The drawing under review shows one solid part. Ordinate dimensions are in mm from its lowest x, y, z. Give positions to 0.01 mm unless a question says otherwise; leave off trailing zeros. Order: outer loops, then holes, each group sorted by start corner. A loop starts at its lowest first (then second) coordinate and runs counter-clockwise, first axis right, second up. Notation, with made-up numbers: (44.25, -21) -> (71.25, -21) arc R32 cw to (71.25, 5) -> close; hole circle Ø11 at (-1.5, 56.5). An arc over 180 degrees is marked (long way). Use CSV: the item, a comma, the result in double quotes. Start each with the question number.
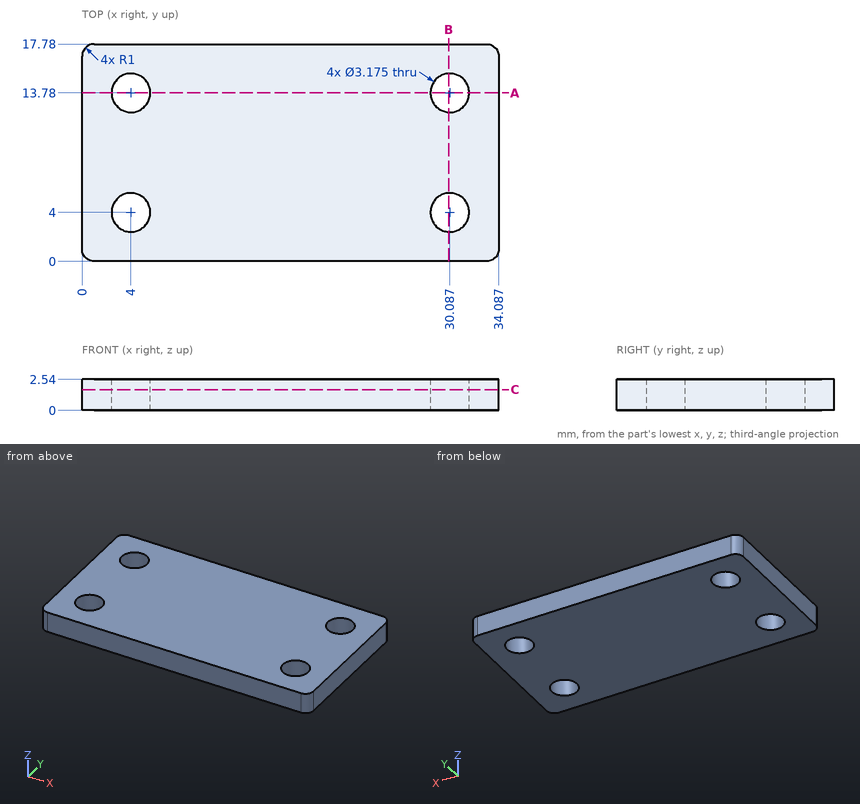
1. To check wall thickness, follow L1, parallel to Y at x = 4, z = 1.5; L2, parallel to Y at x = 5, z = 0.1. State the ranges of each line that lie inside material, in increasing order. Write a range as [from, to].
2. Consider section C-C (z = 1.7). State the section outline as (x, y) points (1 decimal).
3. Consider section A-A (y = 13.78). State the section outline as (x, z) points.
4. Consider section B-B (x = 30). State the section outline as (y, z) points (1 decimal).
5. Clearance check with flat-ended pins moving along their axes: P1, Ø4, axis at x = 4, y = 4, coming from the +Z side; P2, Ø3, axis at x = 30.09, y = 4, coming from the -Z side. State where each tip first meets the part, or that it passes through.
Answer list:
1,L1,"[0, 2.41], [5.59, 12.19], [15.37, 17.78]"
1,L2,"[0, 2.77], [5.23, 12.55], [15.01, 17.78]"
2,outline,"(0, 1) arc R1 ccw to (1, 0) -> (33.1, 0) arc R1 ccw to (34.1, 1) -> (34.1, 16.8) arc R1 ccw to (33.1, 17.8) -> (1, 17.8) arc R1 ccw to (0, 16.8) -> close; hole circle Ø3.2 at (4, 4); hole circle Ø3.2 at (4, 13.8); hole circle Ø3.2 at (30.1, 4); hole circle Ø3.2 at (30.1, 13.8)"
3,outline,"(0, 0) -> (2.41, 0) -> (2.41, 2.54) -> (0, 2.54) -> close; (5.59, 0) -> (28.5, 0) -> (28.5, 2.54) -> (5.59, 2.54) -> close; (31.67, 0) -> (34.09, 0) -> (34.09, 2.54) -> (31.67, 2.54) -> close"
4,outline,"(0, 0) -> (2.4, 0) -> (2.4, 2.5) -> (0, 2.5) -> close; (5.6, 0) -> (12.2, 0) -> (12.2, 2.5) -> (5.6, 2.5) -> close; (15.4, 0) -> (17.8, 0) -> (17.8, 2.5) -> (15.4, 2.5) -> close"
5,P1,"z = 2.54"
5,P2,"through"
